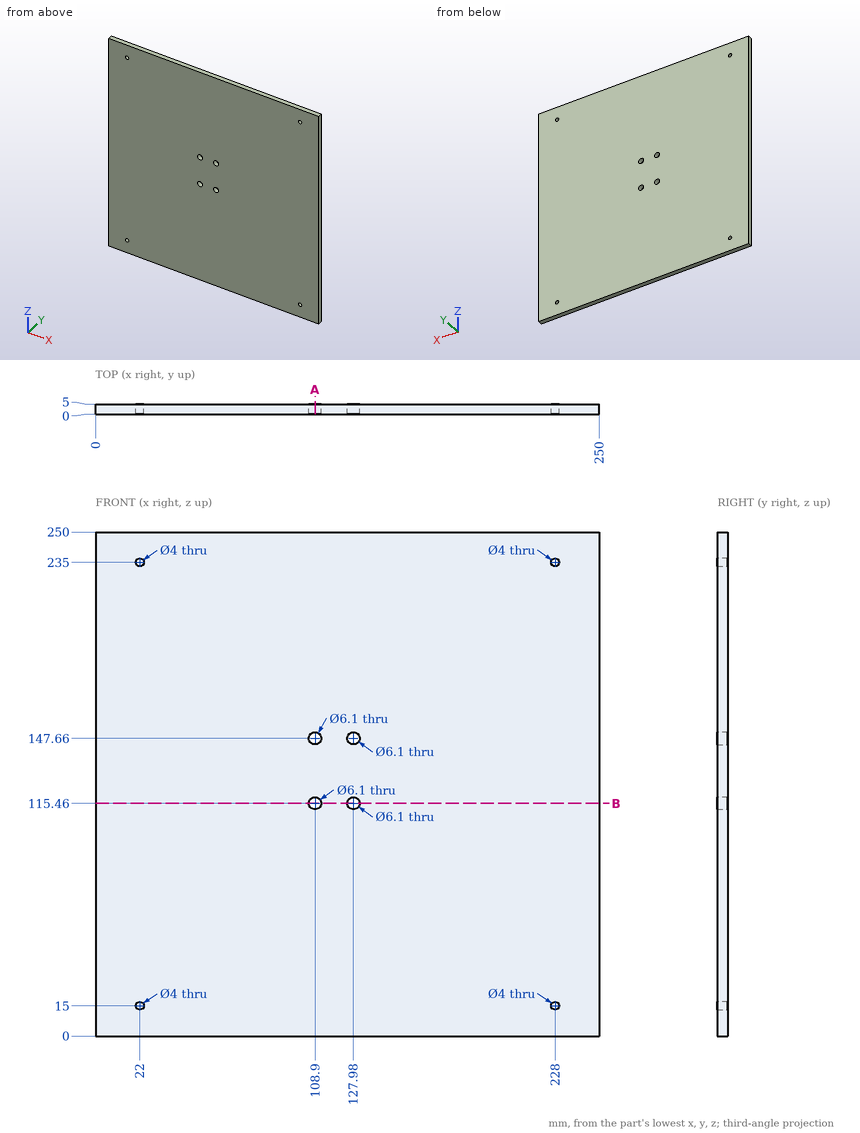
Can you work these out from the drawing? Everything is in mm from the part's minimum corner. Coordinates: 2 decimals unless noted, no trailing zeros. Loops run counter-clockwise (first coordinate to the right, second up) from the corner with the lowest first, then second, coordinate; pieces in that order, holes last.
1) Imagine slicing it at A-A (x = 108.9). List the corners of the cut face in (y, z) for me.
Reported:
outline: (0, 0) - (5, 0) - (5, 112.41) - (0, 112.41) - close; (0, 118.51) - (5, 118.51) - (5, 144.61) - (0, 144.61) - close; (0, 150.71) - (5, 150.71) - (5, 250) - (0, 250) - close
2) Please list where these lines run through material, in increasing order: line 1 along X through (y, z) = (2.5, 115.46); line 2 along Z through (x, y) = (228, 2.45); line 3 along X through (y, z) = (3.2, 235).
Reported:
line 1: x = 0 to 105.85, 111.95 to 124.93, 131.03 to 250
line 2: z = 0 to 13, 17 to 233, 237 to 250
line 3: x = 0 to 20, 24 to 226, 230 to 250
3) Will this pin go through, and if not, where does the flat tip stop? pin 1 Ø3 at (x, z) = (22, 15) entering from -Y.
Reported:
pin 1: passes through
4) Imagine slicing it at B-B (z = 115.46). List the corners of the cut face in (x, y) for me, and give its area (3 significant figures).
Reported:
outline: (0, 0) - (105.85, 0) - (105.85, 5) - (0, 5) - close; (111.95, 0) - (124.93, 0) - (124.93, 5) - (111.95, 5) - close; (131.03, 0) - (250, 0) - (250, 5) - (131.03, 5) - close
area: 1,190 mm2
